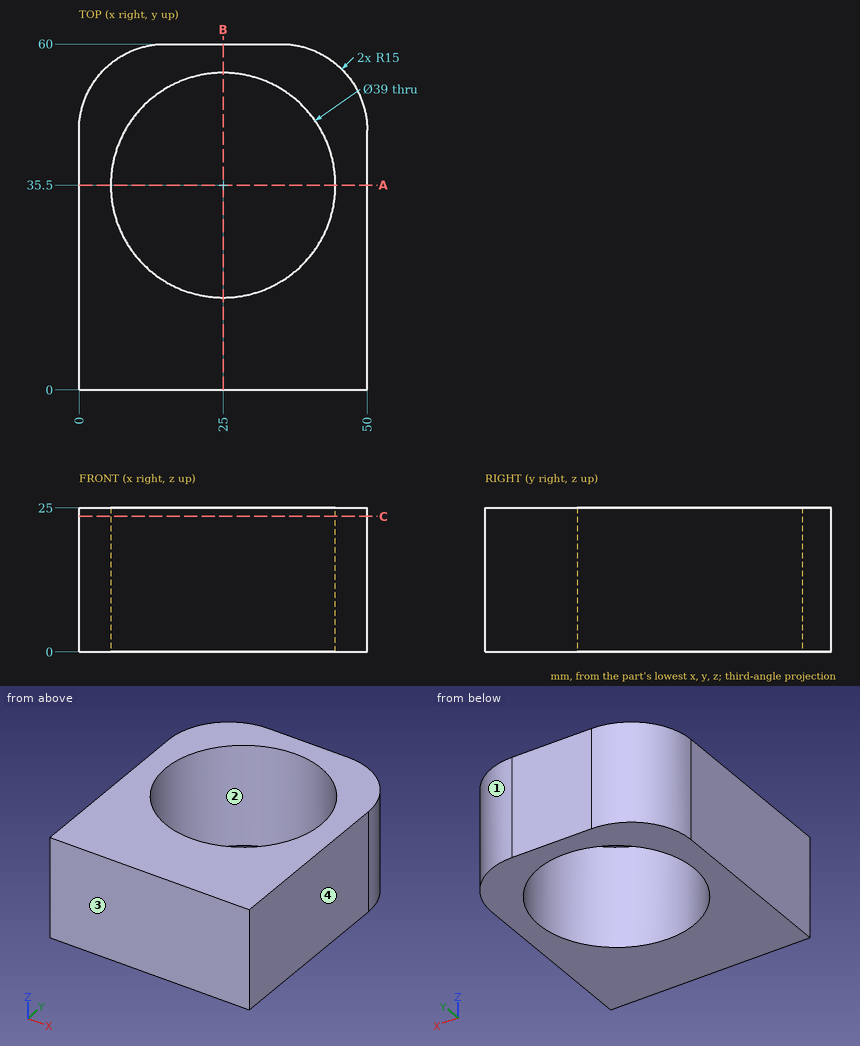
Part print with two shaded views. Sizes in mm from the minimum x, y, z corner. Round coordinates to 2 decimals unless told otherwise and drop trailing zeros. Loops run counter-clockwise (first coordinate to the right, second up) from the corner with the lowest first, then second, coordinate; pieces in that order, holes last. Notation, with made-up numbers: (24.5, -3) - (39.5, -3) arc R9 cw to (39.5, 13) - close; hole circle Ø1 at (89, -6). An arc over 180 degrees is marked (long way). Answer as a JSON object with one key per item and string values.
Item 1: Pull direction Y, two halves, no side cores. Call the marked faces 1, 2, 3 and 4: pulls with the +Y half, pulls with the -Y half, needs draft (parallel to the pull), parting line crosses it, or undercut.
Output:
{"face 1": "pulls with the +Y half", "face 2": "undercut", "face 3": "pulls with the -Y half", "face 4": "needs draft"}
Item 2: Wall check: L1, parallel to Y at x = 25, z = 16; L2, parallel to Y at x = 41, z = 15; L3, parallel to X at y = 46.5, z = 13.5. Give the ranges that are in metal, low to high.
Output:
{"L1": "0 to 16, 55 to 60", "L2": "0 to 24.35, 46.65 to 58.75", "L3": "0.08 to 8.9, 41.1 to 49.92"}
Item 3: Band-saw the part on A-A on y = 35.5. List the corners of the cut face in (x, z).
Output:
{"outline": "(0, 0) - (5.5, 0) - (5.5, 25) - (0, 25) - close; (44.5, 0) - (50, 0) - (50, 25) - (44.5, 25) - close"}
Item 4: Band-saw the part on B-B on x = 25. List the corners of the cut face in (y, z).
Output:
{"outline": "(0, 0) - (16, 0) - (16, 25) - (0, 25) - close; (55, 0) - (60, 0) - (60, 25) - (55, 25) - close"}
Item 5: Pin check, flat tips, straight feed: pin 1 (4 mm diameter, centred on y = 53.5, z = 20.5, fed in from -X); pin 2 (8 mm diameter, centred on x = 9, z = 3.5, fed in from +Y). Stop position of each tip, or through.
Output:
{"pin 1": "x = 1.48", "pin 2": "y = 59.87"}
Item 6: Band-saw the part on C-C on z = 23.5. List the corners of the cut face in (x, y), plus the area to 3 significant figures.
Output:
{"outline": "(0, 0) - (50, 0) - (50, 45) arc R15 ccw to (35, 60) - (15, 60) arc R15 ccw to (0, 45) - close; hole circle Ø39 at (25, 35.5)", "area": "1,710 mm2"}
